Job drawing, mm, ordinate dimensions from the low corner. One solid piece. Give positions to 0.01 mm unless a question says otherwise; leave off trailing zeros. Order: outer loops, then holes, each group sorted by start corner. A loop starts at its lowest first (then second) coordinate and runs counter-clockwise, first axis right, second up. Notation, with made-up numbers: (57, 71.5) - (69, 71.5) arc R16 ccw to (69, 100.5) - close; hole circle Ø10 at (64.5, -3.75). An arc over 180 degrees is marked (long way). One line per item, written item: value.
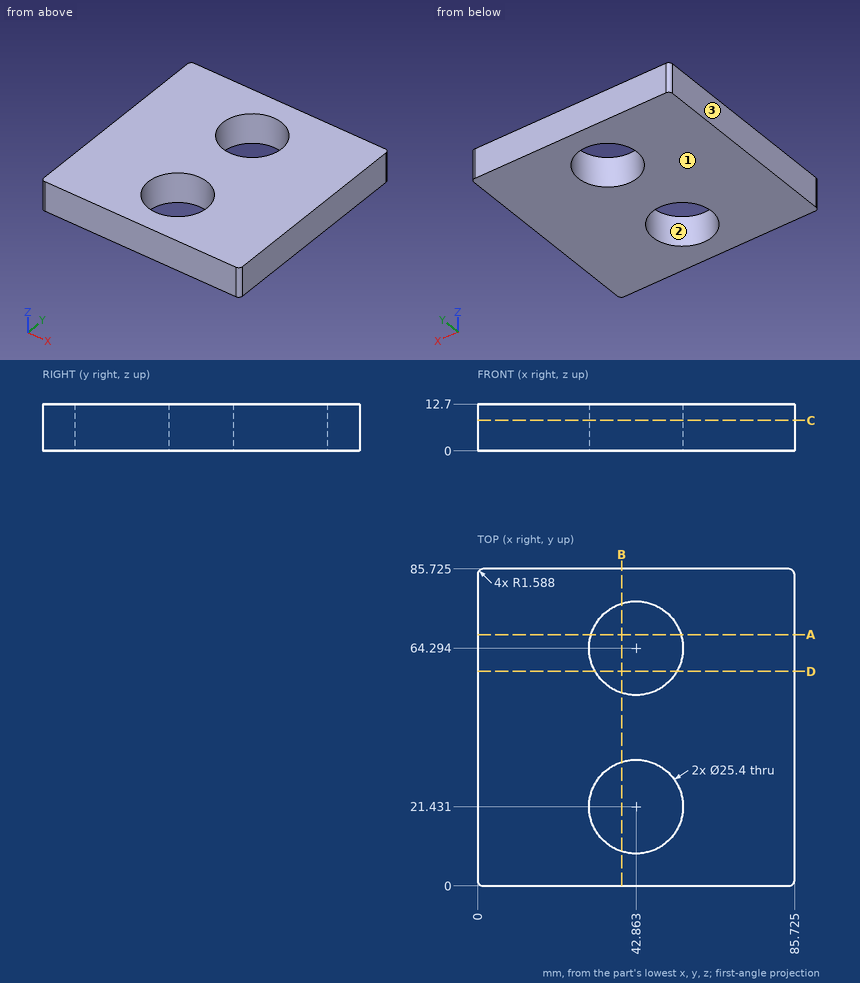
1) Slice it at D-D on y = 58. Write the cut outline in (x, z) (1 decimal).
Answer:
outline: (0, 0) - (31.8, 0) - (31.8, 12.7) - (0, 12.7) - close; (53.9, 0) - (85.7, 0) - (85.7, 12.7) - (53.9, 12.7) - close
2) Drop a flat-ended pin along its axis: P1, Ø6, axis at y = 15.5, z = 5.5, coming from the -X side. Give the stop position or say it passes through.
Answer:
P1: stops at x = 0
3) Two-plate mould, pull along X, no slides. Class the marked faces 1, 2 and 3: pulls with the +X half, pulls with the -X half, needs draft (parallel to the pull), parting line crosses it, or undercut.
Answer:
face 1: needs draft
face 2: undercut
face 3: pulls with the -X half
4) Slice it at B-B on x = 39. Write the cut outline in (y, z) (1 decimal).
Answer:
outline: (0, 0) - (9.3, 0) - (9.3, 12.7) - (0, 12.7) - close; (33.5, 0) - (52.2, 0) - (52.2, 12.7) - (33.5, 12.7) - close; (76.4, 0) - (85.7, 0) - (85.7, 12.7) - (76.4, 12.7) - close
5) Slice it at A-A on y = 68. Write the cut outline in (x, z) (1 decimal).
Answer:
outline: (0, 0) - (30.7, 0) - (30.7, 12.7) - (0, 12.7) - close; (55, 0) - (85.7, 0) - (85.7, 12.7) - (55, 12.7) - close
6) Slice it at C-C on z = 8.25. Write the cut outline in (x, y) (1 decimal).
Answer:
outline: (0, 1.6) arc R1.6 ccw to (1.6, 0) - (84.1, 0) arc R1.6 ccw to (85.7, 1.6) - (85.7, 84.1) arc R1.6 ccw to (84.1, 85.7) - (1.6, 85.7) arc R1.6 ccw to (0, 84.1) - close; hole circle Ø25.4 at (42.9, 21.4); hole circle Ø25.4 at (42.9, 64.3)
7) Wall check: line 1 along Y through (x, z) = (43, 7) (1 decimal); line 2 along Y through (x, z) = (53.5, 7.25) (1 decimal); line 3 along X through (y, z) = (29.5, 10.5) (1 decimal). Give the ranges that are in metal, low to high. Write a range as [from, to].
Answer:
line 1: y = [0, 8.7], [34.1, 51.6], [77, 85.7]
line 2: y = [0, 14.5], [28.4, 57.4], [71.2, 85.7]
line 3: x = [0, 33.1], [52.7, 85.7]
